Verification items for this drawing (mm, ordinates from the low corner). A direction names the side the tool comes from. Give positions to 0.01 mm unless a question says otherwise; leave off trailing zeros. Loops run counter-clockwise (first coordinate to the right, second up) from the corner with the lowest first, then second, coordinate; pieces in that order, holes last. Notation, with made-up numbers: M -38,57.5 L -1,57.5 A24 ccw -1,92.5 Z; hole C 67,70.5 d7. An arc over 180 degrees is marked long. Put each result on its own line as item: value. Start each with the question number.
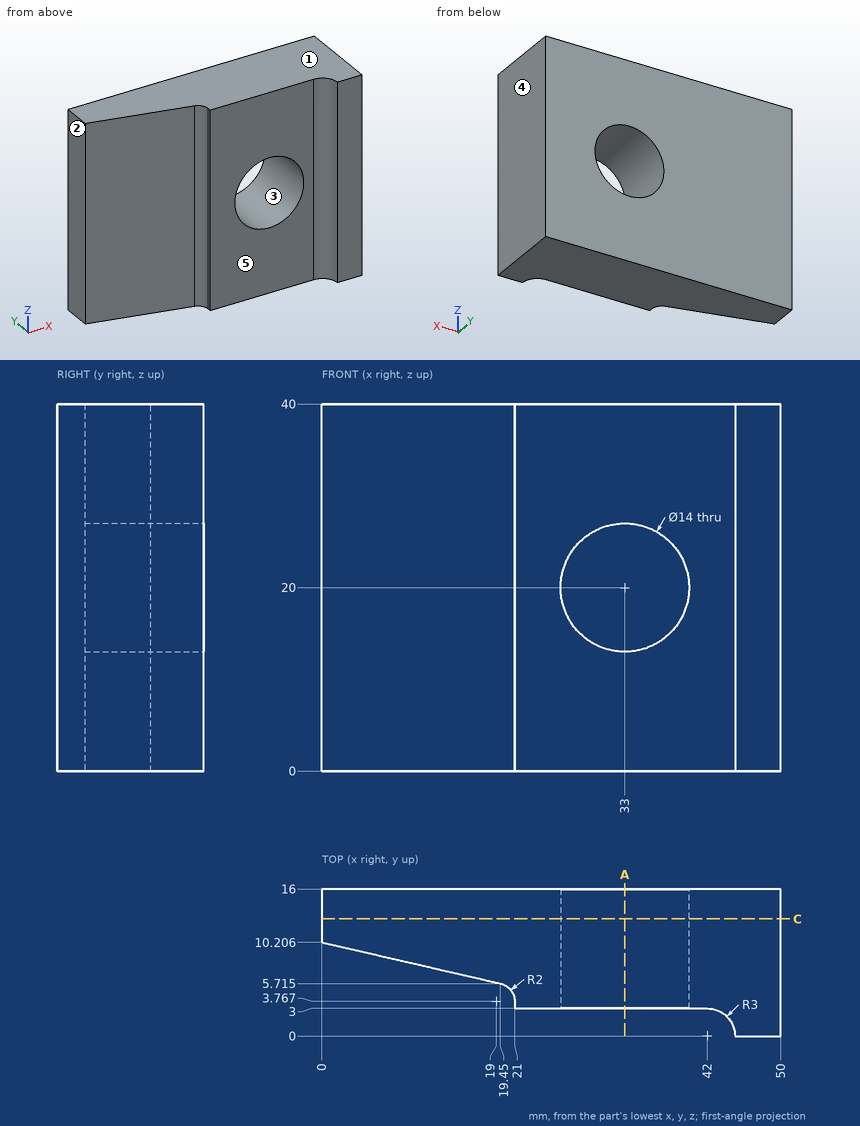
Q1. Release check for a two-part mould opening along X. For the marked faces 1, 2 and 3 record: pulls with the +X half, pulls with the -X half, needs draft (parallel to the pull), parting line crosses it, or undercut.
Q2. Cross-section at C-C, the plane y = 12.75. Record the boundary of the cut face in (x, z).
Q3. Set-up check for the marked faces 4 and 5: record each of +Z, -Z, +X, -X, +Y, -Y from which the full face is reachable in a straight line by a thin tool's end or side.
Q4. Scan lines: L1, parallel to Z at x = 33, y = 7; L2, parallel to Z at x = 30, y = 6.5 (1 decimal); L3, parallel to Y at x = 32, z = 32.5. Record each from-to range of solid material in increasing order.
Q5. Cross-section at A-A, the plane x = 33. Record the boundary of the cut face in (y, z), then the cut area to 3 significant figures.
Q6. Go/stop test with flat-tipped pins: pin 1 (5 mm diameter, centred on x = 29.5, y = 10, fed in from -Z); pin 2 (0.6 mm diameter, centred on y = 3.5, z = 16.5, fed in from -X); pin 3 (1.5 mm diameter, centred on y = 4.5, z = 22.5, fed in from -X). Record where each tip stops, or that it passes through.
Ans:
1. face 1: needs draft
1. face 2: pulls with the -X half
1. face 3: undercut
2. outline: M 0,0 L 50,0 L 50,40 L 0,40 Z; hole C 33,20 d14
3. face 4: +Z, -Z, +X, +Y, -Y
3. face 5: +Z, -Z, -X, -Y
4. L1: z = 0 to 13, 27 to 40
4. L2: z = 0 to 13.7, 26.3 to 40
4. L3: y = 3 to 16
5. outline: M 3,0 L 16,0 L 16,13 L 3,13 Z; M 3,27 L 16,27 L 16,40 L 3,40 Z
5. area: 338 mm^2
6. pin 1: stops at z = 0
6. pin 2: stops at x = 21
6. pin 3: stops at x = 20.34
